Design review of the part built by this model. Coordinates are the model's own, in mm. Give positions to 0.01 mm unless a question says otherwise; leave off trailing zeros. Write each loop counter-clockwise with the first axis right and the second up, starting at its lowest first coordinate (ties: lowest second). Pieces come first, ordered by that corner, then holes. Notation, with made-up numbers: M 29.25,13 L 46.25,13 A32 ccw 46.25,50 Z; hole C 84.25,-9.75 d8. An arc over 180 degrees is marked long. Answer in a Markdown table with one row per item.
```python
from build123d import *

# Parameters (mm, degrees)
BOSS_EXTRUDE1_DEPTH  = 1.5875
M8_CLEARANCE_HOLE1_D = 8.4


with BuildPart() as part:
    # Sketch1 → Boss-Extrude1 (new body)
    with BuildSketch(Plane(origin=(0, 0, 0), x_dir=(0, 0, -1), z_dir=(1, 0, 0))):
        with BuildLine():
            Line((-14.2875, -118.025122157), (0, -118.025122157))
            Line((0, -118.025122157), (14.2875, -118.025122157))
            Line((14.2875, -118.025122157), (10.667522727, -28.168425744))
            Line((10.667522727, -28.168425744), (9.081309394, -28.232328118))
            Line((9.081309394, -28.232328118), (8.442285655, -12.370194791))
            Line((8.442285655, -12.370194791), (10.028498987, -12.306292417))
            Line((10.028498987, -12.306292417), (9.517279996, 0.383414244))
            ThreePointArc((9.517279996, 0.383414244), (0, 9.525), (-9.517279996, 0.383414244))
            Line((-9.517279996, 0.383414244), (-10.028498987, -12.306292417))
            Line((-10.028498987, -12.306292417), (-8.442285655, -12.370194791))
            Line((-8.442285655, -12.370194791), (-9.081309394, -28.232328118))
            Line((-9.081309394, -28.232328118), (-10.667522727, -28.168425744))
            Line((-10.667522727, -28.168425744), (-14.2875, -118.025122157))
        make_face()
    extrude(amount=BOSS_EXTRUDE1_DEPTH)

    # M8 Clearance Hole1 (through all)
    with Locations(Plane(origin=(1.5875, 0, 0), x_dir=(0, 0, -1), z_dir=(1, 0, 0))):
        with Locations((0, 0)):
            Hole(M8_CLEARANCE_HOLE1_D / 2)


solid = part.part
```
1) Add section C-C (y = -74). Write out the cut boundary in (x, z), and give its area (3 significant figures).
Geometry says:
| item | result |
|---|---|
| outline | M 0,-12.51 L 1.59,-12.51 L 1.59,12.51 L 0,12.51 Z |
| area | 39.7 mm^2 |
2) The part is to be moulded in two halves that separate along Z. For faces 1 (the face through (0.783, -72.468, 12.452)), 2 (the face through (0.783, 9.523, -0.204)), 3 (the face through (0, -68, 0)), 4 (the face through (0.783, 1.262, 4.006)), say which applies: released by +Z, released by -Z, zero draft, split by the parting line, or undercut.
Geometry says:
| item | result |
|---|---|
| face 1 | released by +Z |
| face 2 | split by the parting line |
| face 3 | zero draft |
| face 4 | undercut |
3) To check wall thickness, follow probe 1 along Y at (x, z) = (0.45, 0) (3 decimals); probe 2 along Y at (x, z) = (1, -1.75); probe 3 along Z at (x, y) = (1, -85). State the ranges of each line that lie inside material, in increasing order. Write a range as [from, to].
Geometry says:
| item | result |
|---|---|
| probe 1 | [-118.025, -4.2], [4.2, 9.525] |
| probe 2 | [-118.03, -3.82], [3.82, 9.36] |
| probe 3 | [-12.96, 12.96] |
4) Add section B-B (z = 0). Write out the cut boundary in (x, y) (1 decimal).
Geometry says:
| item | result |
|---|---|
| outline | M 0,-118 L 1.6,-118 L 1.6,-4.2 L 0,-4.2 Z; M 0,4.2 L 1.6,4.2 L 1.6,9.5 L 0,9.5 Z |
5) Add section D-D (z = -12). Write out the cut boundary in (x, y), and give its area (3 significant figures).
Geometry says:
| item | result |
|---|---|
| outline | M 0,-118.03 L 1.59,-118.03 L 1.59,-61.24 L 0,-61.24 Z |
| area | 90.1 mm^2 |
6) Insertion check: P1, Ø13.5, axis at y = 0, z = 0, coming from the +X side. The pin has a flat end and moves straight along its axis. Give the tip position at first contact, or say it passes through.
Geometry says:
| item | result |
|---|---|
| P1 | x = 1.59 |
